The listing builds one solid part. Answer for the finished solid, in the listing's coordinates (mm). Coordinates: 2 decimals unless noted, no trailing zeros. Order: outer loops, then holes, each group sorted by start corner. A loop starts at its lowest first (then second) coordinate and runs counter-clockwise, first axis right, second up. Notation, with made-up numbers: (54.25, -23) -> (99.25, -23) arc R16 ccw to (99.25, 1) -> close; hole circle Ø2 at (41.25, 82). An arc over 180 degrees is marked (long way). One line per question, with ' | ' between items.
from build123d import *

# Parameters (mm, degrees)
BLANKSKE_W               = 60
BLANKSKE_H               = 5.8
BLANK_DEPTH              = 2.5
TOOTHCUTSIM_DEPTH        = 61.331500893
TEETHCUTS_COUNT          = 25
TEETHCUTS_PITCH          = 2.51327412
EXTRUDE_1_DEPTH          = 2.5
SKETCH_3_R               = 1.45
CUT_EXTRUDE_1_DEPTH      = 23
CUT_EXTRUDE_1_DEPTH_BACK = 12


with BuildPart() as part:
    # BlankSke → Blank (new body)
    with BuildSketch(Plane.XY):
        with Locations((30, 2.9)):
            Rectangle(BLANKSKE_W, BLANKSKE_H)
    extrude(amount=-BLANK_DEPTH)

    # TooCutSkeSim → ToothCutSim (cut, through all)
    with BuildSketch(Plane.XY):
        Polygon((0.354348296, 4), (-0.354348296, 4), (-1.018739561, 5.8254), (1.018739561, 5.8254), align=None)
    toothcutsim = extrude(amount=-TOOTHCUTSIM_DEPTH, mode=Mode.SUBTRACT)

    # TeethCuts: ToothCutSim ×25
    with Locations(*[(i * TEETHCUTS_PITCH, 0, 0) for i in range(1, TEETHCUTS_COUNT)]):
        add(toothcutsim, mode=Mode.SUBTRACT)

    # 草图2 → 凸台-拉伸1 (add)
    with BuildSketch(Plane(origin=(0, 0, -2.5), x_dir=(-1, 0, 0), z_dir=(0, 0, -1))):
        Polygon((0, 4), (0, -4), (-12, -4), (-18.92820323, 0), align=None)
    extrude(amount=-EXTRUDE_1_DEPTH)

    # 草图3 → 切除-拉伸1 (cut, two sides)
    with BuildSketch(Plane(origin=(0, 0, -2.5), x_dir=(-1, 0, 0), z_dir=(0, 0, -1))) as cut_extrude_1_sk:
        with Locations((-3, 0.5)):
            Circle(SKETCH_3_R)
        with Locations((-13.794228634, 0.5)):
            Circle(SKETCH_3_R)
    extrude(amount=CUT_EXTRUDE_1_DEPTH, mode=Mode.SUBTRACT)
    extrude(cut_extrude_1_sk.sketch, amount=-CUT_EXTRUDE_1_DEPTH_BACK, mode=Mode.SUBTRACT)


solid = part.part
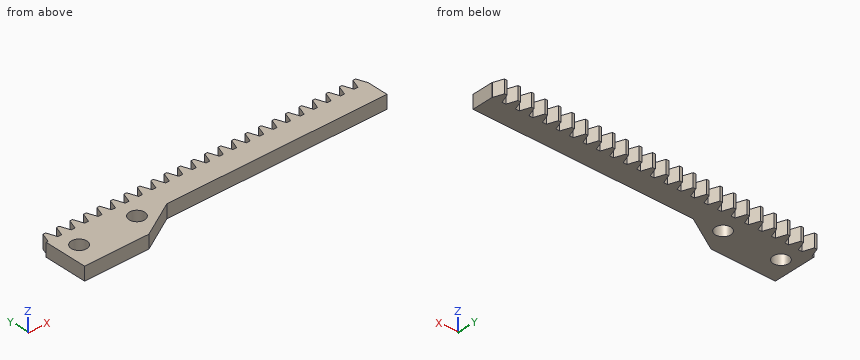
Item 1: Section B-B, the plane z = -1.3 is taken. Count the separate pieces of the cut face and the enclosed holes in it, plus the area to 3 significant figures.
Computed values:
separate pieces: 1 | enclosed holes: 2 | area: 338 mm^2
Item 2: Section A-A, the plane y = 0.5 is taken. Give the vertices of the cut face in (x, z).
Computed values:
outline: (0, -2.5) -> (1.55, -2.5) -> (1.55, 0) -> (0, 0) -> close; (4.45, -2.5) -> (12.34, -2.5) -> (12.34, 0) -> (4.45, 0) -> close; (15.24, -2.5) -> (60, -2.5) -> (60, 0) -> (15.24, 0) -> close
Item 3: Find the intervals of material crossed by L1, parallel to X at y = 1.25, z = -0.9; L2, parallel to Y at x = 33, z = -0.5; L3, parallel to X at y = -0.25, z = -1.65, in increasing order.
Computed values:
L1: x = 0 to 1.76, 4.24 to 12.55, 15.04 to 60 | L2: y = 0 to 4 | L3: x = 0 to 1.76, 4.24 to 12.55, 15.04 to 18.5
